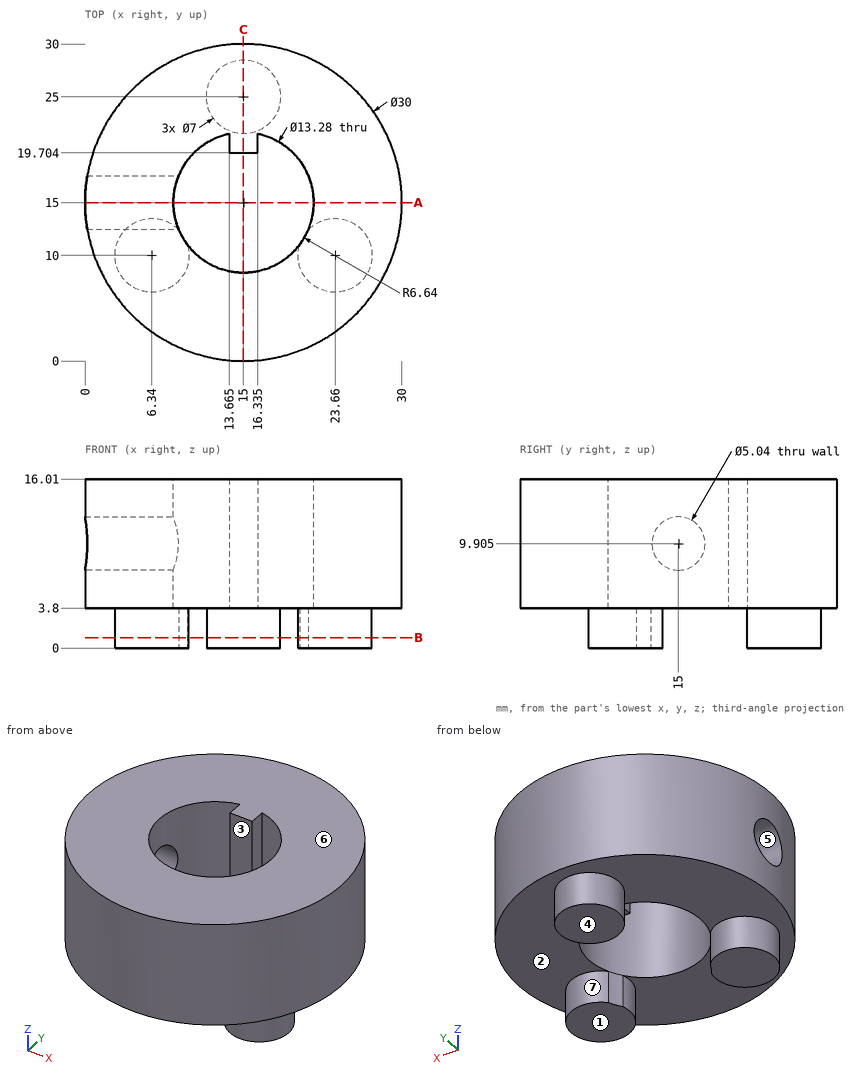
Study the drawing (mm; zero at the part's minimum x, y, z) and answer. A direction names the side the tool comes from. Round coordinates to 2 decimals unless told otherwise and drop trailing zeros. Loops run counter-clockwise (first coordinate to the right, second up) from the corner with the lowest first, then second, coordinate; pieces in that order, holes last.
Q1. Section B-B, the plane z = 1 is taken. Determine the outline of the cut face in (x, y) (1 decimal), then the cut area to 3 significant figures.
Q2. Given pin 1 Ø1 at (y, z) = (24.5, 5) entering from -X; pin 2 Ø1 at (y, z) = (10, 4.5) entering from +X; pin 3 Ø8 at (y, z) = (5.5, 12) entering from +X (1 decimal), each flat-ended and moving along its own axis, determine where each tip first touches the part or whether it passes through.
Q3. Section A-A, the plane y = 15 is taken. Determine the outline of the cut face in (x, z) (1 decimal).
Q4. For a pull along Z with two mould halves and no side action, classify the marked faces 4, 5, 6 and 7 as released by +Z, released by -Z, zero draft, split by the parting line, or undercut.
Q5. Which of the six approach directions +Z, -Z, +X, -X, +Y, -Y give full straight-line access (tool end or side, diameter ignored) to the marked faces 1, 2 and 3?
Q6. Find the intervals of material crossed by line 1 (Z direction, x = 17, y = 21.5); line 2 (X direction, y = 12, z = 11) (1 decimal); line 3 (Z direction, x = 8.5, y = 17), in increasing order.
Q7. Section C-C, the plane x = 15 is taken. Determine the outline of the cut face in (y, z) (1 decimal), then the cut area to 3 significant figures.
Completed:
1. outline: (8.9, 12.4) arc R3.5 ccw (long way) to (9.7, 11) arc R6.6 cw to start; circle Ø7 at (15, 25); (20.3, 11) arc R3.5 ccw (long way) to (21.1, 12.4) arc R6.6 cw to start
1. area: 115 mm2
2. pin 1: stops at x = 3
2. pin 2: stops at x = 29.31
2. pin 3: stops at x = 29
3. outline: (0, 3.8) - (8.4, 3.8) - (8.4, 7.4) - (0, 7.4) - close; (0, 12.4) - (8.4, 12.4) - (8.4, 16) - (0, 16) - close; (21.6, 3.8) - (30, 3.8) - (30, 16) - (21.6, 16) - close
4. face 4: released by -Z
4. face 5: undercut
4. face 6: released by +Z
4. face 7: zero draft
5. face 1: -Z, +X, -X, +Y, -Y
5. face 2: -Z
5. face 3: +Z, -Z
6. line 1: z = 3.8 to 16.01
6. line 2: x = 0.3 to 9.1, 20.9 to 29.7
6. line 3: z = 3.8 to 8.37, 11.44 to 16.01
7. outline: (0, 3.8) - (8.4, 3.8) - (8.4, 16) - (0, 16) - close; (19.7, 3.8) - (21.5, 3.8) - (21.5, 0) - (28.5, 0) - (28.5, 3.8) - (30, 3.8) - (30, 16) - (19.7, 16) - close
7. area: 254 mm2
